Answer from the drawing. Dimensions are ordinates in mm from the lowest x, y and z of the part. Give positions to 0.01 mm unless a question says otherwise; leave off trailing zeros. Loops run counter-clockwise (first coordinate to the right, second up) from the corner with the lowest first, then second, coordinate; pieces in that order, holes last. Notation, with made-up numbers: (61, 52) -> (88, 52) arc R32 cw to (88, 85) -> close; hole circle Ø1 at (8, -38). An arc over 180 degrees is marked (long way). Write each question's results on one line, items separated by ' | '. Start each with the question number.
Item 1: Section D-D on y = 0.85 is taken. Write down the section's boundary in (x, z), and give its area (3 significant figures).
Item 2: This flat-tipped pin is pushed along its axis until it touches: P1, Ø0.6, axis at x = 17.5, y = 0.5, coming from the +Z side. Where does it stop, or does it pass through?
Item 3: Section A-A on z = 5 is taken. Write down the section's boundary in (x, y), and give its area (3 significant figures).
Item 4: Find the intervals of material crossed by line 1 (Z direction, x = 35, y = 0.95); line 2 (Z direction, x = 10, y = 0.35); line 3 (Z direction, x = 25, y = 0.9), in increasing order.
Item 5: Section B-B on z = 30 is taken. Write down the section's boundary in (x, y).
Item 6: Section C-C on x = 24 is taken. Write down the section's boundary in (y, z), and give its area (3 significant figures).
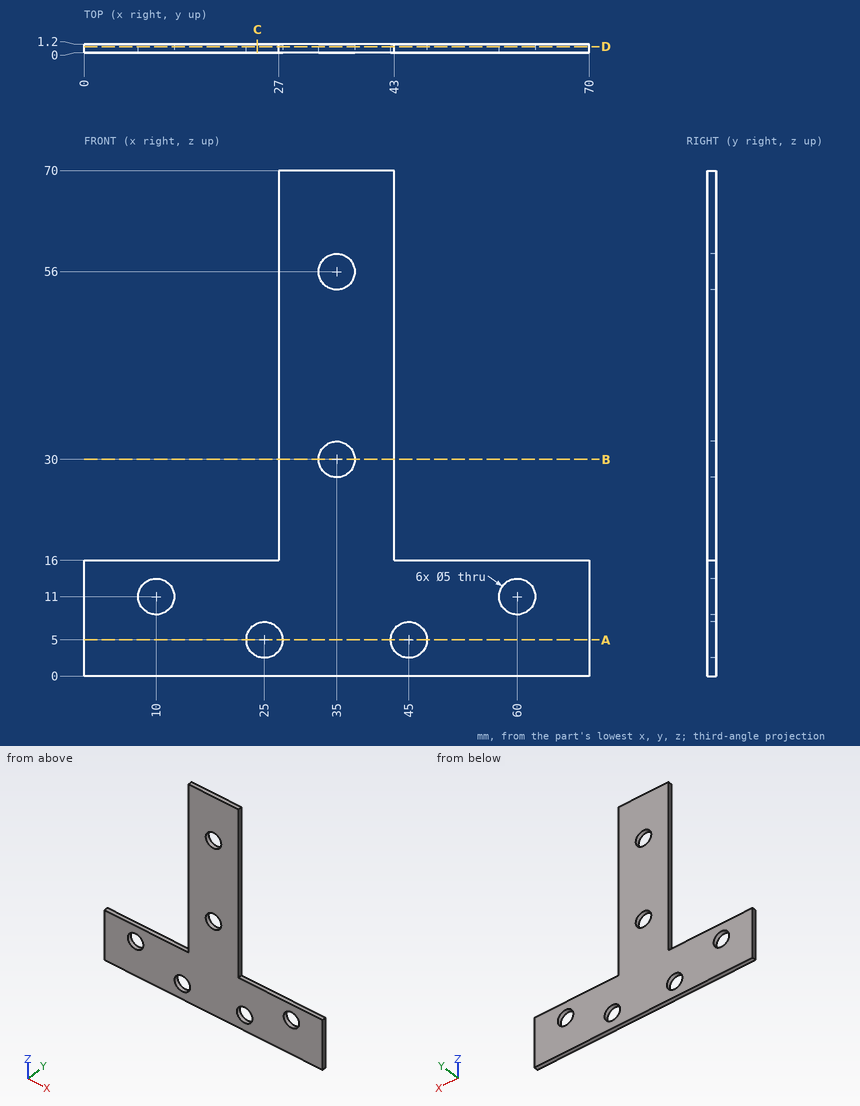
Findings:
1) outline: (0, 0) -> (70, 0) -> (70, 16) -> (43, 16) -> (43, 70) -> (27, 70) -> (27, 16) -> (0, 16) -> close; hole circle Ø5 at (10, 11); hole circle Ø5 at (25, 5); hole circle Ø5 at (35, 30); hole circle Ø5 at (35, 56); hole circle Ø5 at (45, 5); hole circle Ø5 at (60, 11) | area: 1,870 mm2
2) P1: z = 16
3) outline: (0, 0) -> (22.5, 0) -> (22.5, 1.2) -> (0, 1.2) -> close; (27.5, 0) -> (42.5, 0) -> (42.5, 1.2) -> (27.5, 1.2) -> close; (47.5, 0) -> (70, 0) -> (70, 1.2) -> (47.5, 1.2) -> close | area: 72.0 mm2
4) line 1: 0 to 27.5, 32.5 to 53.5, 58.5 to 70 | line 2: 0 to 8.5, 13.5 to 16 | line 3: 0 to 2.5, 7.5 to 16
5) outline: (27, 0) -> (32.5, 0) -> (32.5, 1.2) -> (27, 1.2) -> close; (37.5, 0) -> (43, 0) -> (43, 1.2) -> (37.5, 1.2) -> close
6) outline: (0, 0) -> (1.2, 0) -> (1.2, 2.71) -> (0, 2.71) -> close; (0, 7.29) -> (1.2, 7.29) -> (1.2, 16) -> (0, 16) -> close | area: 13.7 mm2
